```python
from build123d import *

# Parameters (mm, degrees)
EXTRUDE_1_DEPTH     = 4
CUT_EXTRUDE_1_DEPTH = 3
SKETCH_5_R          = 1.25
CUT_EXTRUDE_2_DEPTH = 12.4
SKETCH_6_W          = 17
SKETCH_6_H          = 35
EXTRUDE_2_DEPTH     = 4
SKETCH_7_W          = 13
SKETCH_7_H          = 23
CUT_EXTRUDE_3_DEPTH = 12.1
SKETCH_8_W          = 4
SKETCH_8_H          = 4
SKETCH_8_R          = 1.25
EXTRUDE_3_DEPTH     = 18


with BuildPart() as part:
    # 草圖1 → 填料-伸長1 (new body)
    with BuildSketch(Plane.XY):
        with BuildLine():
            Line((7.5, 0), (7.5, 52))
            ThreePointArc((7.5, 52), (0, 59.5), (-7.5, 52))
            Line((-7.5, 52), (-7.5, 0))
            Line((-7.5, 0), (7.5, 0))
        make_face()
    extrude(amount=EXTRUDE_1_DEPTH)

    # 草圖3 → 除料-伸長1 (cut)
    with BuildSketch(Plane.XY):
        with BuildLine():
            ThreePointArc((-2.5, 48.75876512), (0, 51.25876512), (2.5, 48.75876512))
            Line((2.5, 48.75876512), (5, 33.5))
            Line((5, 33.5), (2.467939071, 17.842139978))
            ThreePointArc((2.467939071, 17.842139978), (-0.200190311, 15.749263002), (-2.5, 18.24123488))
            Line((-2.5, 18.24123488), (-5, 33.5))
            Line((-5, 33.5), (-2.5, 48.75876512))
        make_face()
    extrude(amount=CUT_EXTRUDE_1_DEPTH, mode=Mode.SUBTRACT)

    # 草圖5 → 除料-伸長2 (cut)
    with BuildSketch(Plane.XY):
        with Locations((0, 33.5)):
            Circle(SKETCH_5_R)
    extrude(amount=CUT_EXTRUDE_2_DEPTH, mode=Mode.SUBTRACT)

    # 草圖6 → 填料-伸長2 (add)
    with BuildSketch(Plane.XY):
        with Locations((0, -17.5)):
            Rectangle(SKETCH_6_W, SKETCH_6_H)
    extrude(amount=EXTRUDE_2_DEPTH)

    # 草圖7 → 除料-伸長3 (cut)
    with BuildSketch(Plane.XY):
        with Locations((0, -17.5)):
            Rectangle(SKETCH_7_W, SKETCH_7_H)
    extrude(amount=CUT_EXTRUDE_3_DEPTH, mode=Mode.SUBTRACT)

    # 草圖8 → 填料-伸長3 (add)
    with BuildSketch(Plane.XY):
        with Locations((0, -4)):
            Rectangle(SKETCH_8_W, SKETCH_8_H)
        with Locations((0, -4)):
            Circle(SKETCH_8_R, mode=Mode.SUBTRACT)
        with Locations((0, -31)):
            Rectangle(SKETCH_8_W, SKETCH_8_H)
        with Locations((0, -31)):
            Circle(SKETCH_8_R, mode=Mode.SUBTRACT)
    extrude(amount=-EXTRUDE_3_DEPTH)


solid = part.part
```
Can you work these out from the model? Positions are in its coordinate system, mm. A direction names the side the tool comes from. Coordinates: 2 decimals unless noted, no trailing zeros. Order: outer loops, then holes, each group sorted by start corner. A loop starts at its lowest first (then second) coordinate and runs counter-clockwise, first axis right, second up. Notation, with made-up numbers: (68, 13) -> (93, 13) arc R22 cw to (93, 37) -> close; hole circle Ø10 at (-9.5, 47). An arc over 180 degrees is marked (long way). Write each question's results on one line, items separated by ' | '.
Item 1: If we mould it in two halves opening along X, with no side actions, what happens to faces 4 (the face through (6.5, -18, 2)), 5 (the face through (8.5, -18, 2)), 6 (the face through (-2, -31, -9))? For each: +X half, -X half, draft (parallel to the pull), parting line (faces both ways), or undercut.
Results are:
face 4: undercut | face 5: +X half | face 6: -X half
Item 2: I want a section at D-D, the plane x = 3.5. Write out the boundary of the cut face in (y, z), then the cut area to 3 significant figures.
Results are:
outline: (-35, 0) -> (-29, 0) -> (-29, 4) -> (-35, 4) -> close; (-6, 0) -> (24.22, 0) -> (24.22, 3) -> (42.66, 3) -> (42.66, 0) -> (58.63, 0) -> (58.63, 4) -> (-6, 4) -> close | area: 227 mm²
Item 3: I'm going to push flat-ended pins straight in: pin 1 Ø2 at (y, z) = (-5, -5) entering from +X; pin 2 Ø10 at (y, z) = (19.5, 1.5) entering from -X; pin 3 Ø0.8 at (x, y) = (-0.5, -4) entering from -Z. Where does each tip first touch, or does it pass through?
Results are:
pin 1: x = 2 | pin 2: x = -7.5 | pin 3: z = 0
Item 4: I want a section at B-B, the plane x = 0. Write out the boundary of the cut face in (y, z), then the cut area to 3 significant figures.
Results are:
outline: (-35, 0) -> (-33, 0) -> (-33, -18) -> (-32.25, -18) -> (-32.25, 0) -> (-29.75, 0) -> (-29.75, -18) -> (-29, -18) -> (-29, 4) -> (-35, 4) -> close; (-6, -18) -> (-5.25, -18) -> (-5.25, 0) -> (-2.75, 0) -> (-2.75, -18) -> (-2, -18) -> (-2, 0) -> (15.74, 0) -> (15.74, 3) -> (32.25, 3) -> (32.25, 4) -> (-6, 4) -> close; (34.75, 3) -> (51.26, 3) -> (51.26, 0) -> (59.5, 0) -> (59.5, 4) -> (34.75, 4) -> close | area: 231 mm²
Item 5: I want a section at A-A, the plane z = -4. Write out the boundary of the cut face in (x, y), then the cut area to 3 significant figures.
Results are:
outline: (-2, -33) -> (2, -33) -> (2, -29) -> (-2, -29) -> close; (-2, -6) -> (2, -6) -> (2, -2) -> (-2, -2) -> close; hole circle Ø2.5 at (0, -31); hole circle Ø2.5 at (0, -4) | area: 22.2 mm²
Item 6: I want a section at C-C, the plane y = -4. Write out the boundary of the cut face in (x, z), then the cut area to 3 significant figures.
Results are:
outline: (-8.5, 0) -> (-2, 0) -> (-2, -18) -> (-1.25, -18) -> (-1.25, 0) -> (1.25, 0) -> (1.25, -18) -> (2, -18) -> (2, 0) -> (8.5, 0) -> (8.5, 4) -> (-8.5, 4) -> close | area: 95.0 mm²
Item 7: If I drill on line 1 along Y through (x, z) = (0, 3.4); line 2 along Y through (x, z) = (0.75, -13); line 3 along Y through (x, z) = (0, -7), over which ranges is the centre line in solid material (lowest first)?
Results are:
line 1: -35 to -29, -6 to 32.25, 34.75 to 59.5 | line 2: -33 to -32, -30 to -29, -6 to -5, -3 to -2 | line 3: -33 to -32.25, -29.75 to -29, -6 to -5.25, -2.75 to -2
Item 8: Which directions (+Z, -Z, +X, -X, +Y, -Y) give clear straight access to the entire face, cutting with the end or side of a thin tool? Please do faces 1 (the face through (3.73, 41.24, 1.48)), 2 (the face through (0, -2, -9)), 3 (the face through (7.5, 26, 2)).
Results are:
face 1: -Z | face 2: -Z, +X, -X, +Y | face 3: +Z, -Z, +X, +Y
